Source: CAD feature listing. Evaluate the final solid. Frame: model axes, mm. Face numbers are marked on the shaded views. A direction names the side the tool comes from. Give positions to 0.01 mm unless a question says otherwise; leave off trailing zeros. Order: outer loops, then holes, each group sorted by start corner. A loop starts at its lowest first (then second) coordinate and runs counter-clockwise, first axis right, second up. Notation, with made-up numbers: (-24.75, 73) - (32.25, 73) arc R13 cw to (32.25, 98) - close; hole circle Ø6 at (65, 72). An arc over 180 degrees is marked (long way). Answer as CSV lines item,"result".
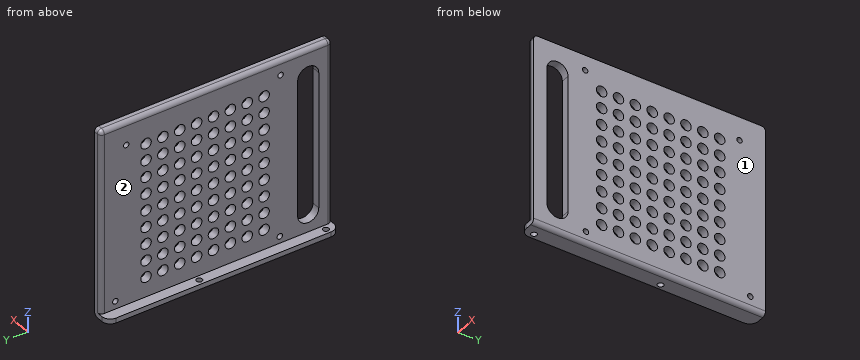
```python
from build123d import *

# Parameters (mm, degrees)
F0_W     = 6.5
F0_H     = 139.7
F0_R     = 1.75
F1_DEPTH = 3
F0_W_2   = 5
F2_DEPTH = 114.3
F3_R     = 1.65
F3_R_2   = 3.175
F4_DEPTH = 25.4
F5_R     = 2.54
F6_R     = 5.08


with BuildPart() as f1:
    # F0 (on Top) → F1 (new body)
    with BuildSketch(Plane.XY):
        with Locations((3.25, 69.85)):
            Rectangle(F0_W, F0_H)
        with Locations((3.25, 5.9583112597)):
            Circle(F0_R, mode=Mode.SUBTRACT)
        with Locations((3.25, 82.1583112597)):
            Circle(F0_R, mode=Mode.SUBTRACT)
    extrude(amount=F1_DEPTH)

    # F0 (on Top) → F2 (join)
    with BuildSketch(Plane.XY):
        with Locations((9, 69.85)):
            Rectangle(F0_W_2, F0_H)
    extrude(amount=F2_DEPTH)

    # F3 (on face) → F4 (cut)
    with BuildSketch(Plane.YZ.offset(11.5)):
        with Locations((31.0318387245, 105.1548512529)):
            Circle(F3_R)
        with Locations((31.5296787245, 7.1532112529)):
            Circle(F3_R)
        with Locations((124.0288587245, 100.2551912529)):
            Circle(F3_R)
        with Locations((130.5287187245, 7.7551912529)):
            Circle(F3_R)
        with Locations((40.965847671, 96.2724089622)):
            Circle(F3_R_2)
        with Locations((40.965847671, 86.1124089622)):
            Circle(F3_R_2)
        with Locations((40.965847671, 75.9524089622)):
            Circle(F3_R_2)
        with Locations((40.965847671, 65.7924089622)):
            Circle(F3_R_2)
        with Locations((40.965847671, 55.6324089622)):
            Circle(F3_R_2)
        with Locations((40.965847671, 45.4724089622)):
            Circle(F3_R_2)
        with Locations((40.965847671, 35.3124089622)):
            Circle(F3_R_2)
        with Locations((40.965847671, 25.1524089622)):
            Circle(F3_R_2)
        with Locations((40.965847671, 14.9924089622)):
            Circle(F3_R_2)
        with Locations((51.125847671, 96.2724089622)):
            Circle(F3_R_2)
        with Locations((51.125847671, 86.1124089622)):
            Circle(F3_R_2)
        with Locations((51.125847671, 75.9524089622)):
            Circle(F3_R_2)
        with Locations((51.125847671, 65.7924089622)):
            Circle(F3_R_2)
        with Locations((51.125847671, 55.6324089622)):
            Circle(F3_R_2)
        with Locations((51.125847671, 45.4724089622)):
            Circle(F3_R_2)
        with Locations((51.125847671, 35.3124089622)):
            Circle(F3_R_2)
        with Locations((51.125847671, 25.1524089622)):
            Circle(F3_R_2)
        with Locations((51.125847671, 14.9924089622)):
            Circle(F3_R_2)
        with Locations((61.285847671, 96.2724089622)):
            Circle(F3_R_2)
        with Locations((61.285847671, 86.1124089622)):
            Circle(F3_R_2)
        with Locations((61.285847671, 75.9524089622)):
            Circle(F3_R_2)
        with Locations((61.285847671, 65.7924089622)):
            Circle(F3_R_2)
        with Locations((61.285847671, 55.6324089622)):
            Circle(F3_R_2)
        with Locations((61.285847671, 45.4724089622)):
            Circle(F3_R_2)
        with Locations((61.285847671, 35.3124089622)):
            Circle(F3_R_2)
        with Locations((61.285847671, 25.1524089622)):
            Circle(F3_R_2)
        with Locations((61.285847671, 14.9924089622)):
            Circle(F3_R_2)
        with Locations((71.445847671, 96.2724089622)):
            Circle(F3_R_2)
        with Locations((71.445847671, 86.1124089622)):
            Circle(F3_R_2)
        with Locations((71.445847671, 75.9524089622)):
            Circle(F3_R_2)
        with Locations((71.445847671, 65.7924089622)):
            Circle(F3_R_2)
        with Locations((71.445847671, 55.6324089622)):
            Circle(F3_R_2)
        with Locations((71.445847671, 45.4724089622)):
            Circle(F3_R_2)
        with Locations((71.445847671, 35.3124089622)):
            Circle(F3_R_2)
        with Locations((71.445847671, 25.1524089622)):
            Circle(F3_R_2)
        with Locations((71.445847671, 14.9924089622)):
            Circle(F3_R_2)
        with Locations((81.605847671, 96.2724089622)):
            Circle(F3_R_2)
        with Locations((81.605847671, 86.1124089622)):
            Circle(F3_R_2)
        with Locations((81.605847671, 75.9524089622)):
            Circle(F3_R_2)
        with Locations((81.605847671, 65.7924089622)):
            Circle(F3_R_2)
        with Locations((81.605847671, 55.6324089622)):
            Circle(F3_R_2)
        with Locations((81.605847671, 45.4724089622)):
            Circle(F3_R_2)
        with Locations((81.605847671, 35.3124089622)):
            Circle(F3_R_2)
        with Locations((81.605847671, 25.1524089622)):
            Circle(F3_R_2)
        with Locations((81.605847671, 14.9924089622)):
            Circle(F3_R_2)
        with Locations((91.765847671, 96.2724089622)):
            Circle(F3_R_2)
        with Locations((91.765847671, 86.1124089622)):
            Circle(F3_R_2)
        with Locations((91.765847671, 75.9524089622)):
            Circle(F3_R_2)
        with Locations((91.765847671, 65.7924089622)):
            Circle(F3_R_2)
        with Locations((91.765847671, 55.6324089622)):
            Circle(F3_R_2)
        with Locations((91.765847671, 45.4724089622)):
            Circle(F3_R_2)
        with Locations((91.765847671, 35.3124089622)):
            Circle(F3_R_2)
        with Locations((91.765847671, 25.1524089622)):
            Circle(F3_R_2)
        with Locations((91.765847671, 14.9924089622)):
            Circle(F3_R_2)
        with Locations((101.925847671, 96.2724089622)):
            Circle(F3_R_2)
        with Locations((101.925847671, 86.1124089622)):
            Circle(F3_R_2)
        with Locations((101.925847671, 75.9524089622)):
            Circle(F3_R_2)
        with Locations((101.925847671, 65.7924089622)):
            Circle(F3_R_2)
        with Locations((101.925847671, 55.6324089622)):
            Circle(F3_R_2)
        with Locations((101.925847671, 45.4724089622)):
            Circle(F3_R_2)
        with Locations((101.925847671, 35.3124089622)):
            Circle(F3_R_2)
        with Locations((101.925847671, 25.1524089622)):
            Circle(F3_R_2)
        with Locations((101.925847671, 14.9924089622)):
            Circle(F3_R_2)
        with Locations((112.085847671, 96.2724089622)):
            Circle(F3_R_2)
        with Locations((112.085847671, 86.1124089622)):
            Circle(F3_R_2)
        with Locations((112.085847671, 75.9524089622)):
            Circle(F3_R_2)
        with Locations((112.085847671, 65.7924089622)):
            Circle(F3_R_2)
        with Locations((112.085847671, 55.6324089622)):
            Circle(F3_R_2)
        with Locations((112.085847671, 45.4724089622)):
            Circle(F3_R_2)
        with Locations((112.085847671, 35.3124089622)):
            Circle(F3_R_2)
        with Locations((112.085847671, 25.1524089622)):
            Circle(F3_R_2)
        with Locations((112.085847671, 14.9924089622)):
            Circle(F3_R_2)
        with BuildLine():
            ThreePointArc((20.7464011222, 97.3240312529), (14.3964011222, 103.6740312529), (8.0464011222, 97.3240312529))
            Line((8.0464011222, 97.3240312529), (8.0464011222, 14.9840312529))
            ThreePointArc((8.0464011222, 14.9840312529), (14.3964011222, 8.6340312529), (20.7464011222, 14.9840312529))
            Line((20.7464011222, 14.9840312529), (20.7464011222, 97.3240312529))
        make_face()
    extrude(amount=-F4_DEPTH, mode=Mode.SUBTRACT)

    # F5 (call 1 of 2: OpenCascade refuses the feature's edges together)
    f5_edges = [f1.edges().sort_by_distance(p)[0] for p in [
        (11.5, 69.85, 0),
    ]]
    fillet(f5_edges, radius=F5_R)

    # F5#2 (call 2 of 2)
    f5_2_edges = [f1.edges().sort_by_distance(p)[0] for p in [
        (6.5, 69.85, 114.3),
        (6.5, 0, 58.65),
        (6.5, 139.7, 58.65),
        (9, 139.7, 114.3),
        (9, 0, 114.3),
    ]]
    fillet(f5_2_edges, radius=F5_R)

    # F6
    f6_edges = [f1.edges().sort_by_distance(p)[0] for p in [
        (0, 0, 1.5),
        (0, 139.7, 1.5),
    ]]
    fillet(f6_edges, radius=F6_R)


solid = f1.part
```
(1) Cut plane C-C (z = 44). Give the number of separate pieces and of enclosed holes in the cut face, then the cut area to 3 significant figures.
Completed:
separate pieces,"10"
enclosed holes,"0"
area,"407 mm²"
(2) Cut plane A-A (y = 10). Return loops of the section in (x, z).
Completed:
outline,"(0, 0) - (8.96, 0) arc R2.54 ccw to (11.5, 2.54) - (11.5, 10.4) - (6.5, 10.4) - (6.5, 3) - (0, 3) - close; (6.5, 101.91) - (11.5, 101.91) - (11.5, 114.3) - (9.04, 114.3) arc R2.54 ccw to (6.5, 111.76) - close"
(3) Cut plane B-B (x = 3.25). Return loops of the section in (y, z), then the cut area to 3 significant figures.
Completed:
outline,"(0.34, 0) - (4.21, 0) - (4.21, 3) - (0.34, 3) - close; (7.71, 0) - (80.41, 0) - (80.41, 3) - (7.71, 3) - close; (83.91, 0) - (139.36, 0) - (139.36, 3) - (83.91, 3) - close"
area,"396 mm²"
(4) Access query for the marked faces 1 and 2. Directions: +Z, -Z, +X, -X, +Y, -Y. A direction counts if a zero-diameter tool reaches every point of the face in a straight line with its end or side. Return the directions, or none.
Completed:
face 1,"+Z, -Z, +X, +Y, -Y"
face 2,"+Z, -X, +Y, -Y"
(5) Ray query, line 1 (Y direction, x = 9.5, z = 41); line 2 (X direction, y = 125, z = 81); line 3 (Z direction, x = 6, y = 129). Return the intervals inside material, ascending. Write a range as from..to.
Completed:
line 1,"0..8.05, 20.75..139.7"
line 2,"6.5..11.5"
line 3,"0..3"
(6) Contact query for flat-ended pins moving along their axis: pin 1 (6 mm diameter, centred on x = 3, y = 42, fed in from -Z); pin 2 (8.5 mm diameter, centred on y = 71.45, z = 35.31, fed in from -X); pin 3 (1 mm diameter, centred on x = 4.5, y = 73.5, fed in from +Z); pin 4 (5 mm diameter, centred on x = 5.5, y = 31.5, fed in from +Z). Output: stop coordinate, or through.
Completed:
pin 1,"z = 0"
pin 2,"x = 6.5"
pin 3,"z = 3"
pin 4,"z = 114.08"
